from build123d import *

# Parameters (mm, degrees)
BOSS_EXTRUDE1_DEPTH = 3
BOSS_EXTRUDE2_DEPTH = 18
SKETCH3_R           = 12
CUT_EXTRUDE1_DEPTH  = 64.419239983
SKETCH4_R           = 1.6
CUT_EXTRUDE2_DEPTH  = 64.419239983
BOSS_EXTRUDE3_DEPTH = 2
BOSS_EXTRUDE4_DEPTH = 3
SKETCH7_R           = 2.2
CUT_EXTRUDE3_DEPTH  = 63.369864518
SKETCH8_R           = 2.2
CUT_EXTRUDE4_DEPTH  = 63.369864518


with BuildPart() as part:
    # Sketch1 → Boss-Extrude1 (new body)
    with BuildSketch(Plane.XY):
        Polygon((0, -43), (0, 0), (43, 0), (43, -13), (19, -13), (13, -19), (13, -43), align=None)
    extrude(amount=BOSS_EXTRUDE1_DEPTH)

    # Sketch2 → Boss-Extrude2 (add)
    with BuildSketch(Plane.XY.offset(3)):
        Polygon((0, -43), (3, -43), (3, -3), (43, -3), (43, 0), (0, 0), align=None)
    extrude(amount=BOSS_EXTRUDE2_DEPTH)

    # Sketch3 → Cut-Extrude1 (cut, through all)
    with BuildSketch(Plane.XY.offset(3)):
        with Locations((22, -22)):
            Circle(SKETCH3_R)
    extrude(amount=-CUT_EXTRUDE1_DEPTH, mode=Mode.SUBTRACT)

    # Sketch4 → Cut-Extrude2 (cut, through all)
    with BuildSketch(Plane.XY.offset(3)):
        with Locations((6.5, -6.5)):
            Circle(SKETCH4_R)
        with Locations((37.5, -6.5)):
            Circle(SKETCH4_R)
        with Locations((6.5, -37.5)):
            Circle(SKETCH4_R)
    extrude(amount=-CUT_EXTRUDE2_DEPTH, mode=Mode.SUBTRACT)

    # Sketch5 → Boss-Extrude3 (add)
    with BuildSketch(Plane(origin=(43, 0, 0), x_dir=(0, 0, -1), z_dir=(1, 0, 0))):
        Polygon((-3, -10), (-11, -3), (-3, -3), align=None)
    extrude(amount=-BOSS_EXTRUDE3_DEPTH)

    # Sketch6 → Boss-Extrude4 (add)
    with BuildSketch(Plane.XZ.offset(43)):
        Polygon((3, 11), (10, 3), (3, 3), align=None)
    extrude(amount=-BOSS_EXTRUDE4_DEPTH)

    # Sketch7 → Cut-Extrude3 (cut, through all)
    with BuildSketch(Plane.XZ.offset(3)):
        with Locations(Location((13, 11, 0), (0, 0, 270))):
            Circle(SKETCH7_R)
        with Locations(Location((33, 11, 0), (0, 0, 270))):
            Circle(SKETCH7_R)
    extrude(amount=-CUT_EXTRUDE3_DEPTH, mode=Mode.SUBTRACT)

    # Sketch8 → Cut-Extrude4 (cut, through all)
    with BuildSketch(Plane(origin=(3, 0, 0), x_dir=(0, 0, -1), z_dir=(1, 0, 0))):
        with Locations((-11, -33)):
            Circle(SKETCH8_R)
        with Locations((-11, -13)):
            Circle(SKETCH8_R)
    extrude(amount=-CUT_EXTRUDE4_DEPTH, mode=Mode.SUBTRACT)


solid = part.part
Check sheet for the modelled part. Datum: model origin and axes. Units: mm. A direction names the side the tool comes from. Round coordinates to 2 decimals unless told otherwise and drop trailing zeros. Loops run counter-clockwise (first coordinate to the right, second up) from the corner with the lowest first, then second, coordinate; pieces in that order, holes last. Notation, with made-up numbers: (-28, 27) -> (4, 27) arc R32 cw to (4, 58) -> close; hole circle Ø2 at (7.5, -13). An arc over 180 degrees is marked (long way). Put each result on its own line as item: value. Start each with the question number.
1. Section check B-B (z = 2.25). Enter the section's corners in (x, y), plus the area to 3 significant figures.
2. Access from +Z, -Z, +X, -X, +Y, -Y to the whole of each face (thin tool, end or side, straight path). Record for faces 4 (the face through (13, -36, 1)), 5 (the face through (41, -6, 6)), 6 (the face through (42.01, -6.55, 6.94)), 7 (the face through (12.7, -14, 3)).
3. Draft check along Y on faces 1 (the face through (6.45, -41.52, 7.06)), 2 (the face through (37.15, -8.06, 1.52)), 3 (the face through (22, 0, 10)). Enter one of: +Y half, -Y half, draft (parallel to the pull), parting line (faces both ways), or undercut.
4. Section check C-C (x = 37.5). Enter the section's corners in (y, z).
5. Section check D-D (y = -33). Enter the section's corners in (x, z), plus the area to 3 significant figures.
6. Scan lines: probe 1 along Y at (x, z) = (1.3, 11); probe 2 along Y at (x, z) = (37.5, 1.9); probe 3 along X at (y, z) = (-5.5, 8). Record each from-to range of solid material in increasing order.
7. Gauge pin test, flat ends, axial feed: pin 1 (9 mm diameter, centred on x = 22.5, z = 9.5, fed in from -Y); pin 2 (0.9 mm diameter, centred on y = -36, z = 1, fed in from +X); pin 3 (3.5 mm diameter, centred on x = 6.5, y = -37.5, fed in from +Z). Record the tip position at first contact, or that the pin passes through.
8. Section check A-A (y = -6.5). Enter the section's corners in (x, z), plus the area to 3 significant figures.
Findings:
1. outline: (0, -43) -> (13, -43) -> (13, -29.94) arc R12 cw to (29.94, -13) -> (43, -13) -> (43, 0) -> (0, 0) -> close; hole circle Ø3.2 at (6.5, -37.5); hole circle Ø3.2 at (6.5, -6.5); hole circle Ø3.2 at (37.5, -6.5)
1. area: 860 mm^2
2. face 4: +Z, -Z, +X, -Y
2. face 5: +Z, -Y
2. face 6: +Z, +X, -Y
2. face 7: +Z
3. face 1: draft
3. face 2: undercut
3. face 3: +Y half
4. outline: (-13, 0) -> (-8.1, 0) -> (-8.1, 3) -> (-13, 3) -> close; (-4.9, 0) -> (0, 0) -> (0, 21) -> (-3, 21) -> (-3, 3) -> (-4.9, 3) -> close
5. outline: (0, 0) -> (13, 0) -> (13, 3) -> (3, 3) -> (3, 8.8) -> (0, 8.8) -> close; (0, 13.2) -> (3, 13.2) -> (3, 21) -> (0, 21) -> close
5. area: 79.8 mm^2
6. probe 1: y = -43 to -35.2, -30.8 to -15.2, -10.8 to 0
6. probe 2: y = -13 to -8.1, -4.9 to 0
6. probe 3: x = 0 to 3, 41 to 43
7. pin 1: stops at y = -3
7. pin 2: stops at x = 13
7. pin 3: stops at z = 3
8. outline: (0, 0) -> (4.9, 0) -> (4.9, 3) -> (3, 3) -> (3, 21) -> (0, 21) -> close; (8.1, 0) -> (35.9, 0) -> (35.9, 3) -> (8.1, 3) -> close; (39.1, 0) -> (43, 0) -> (43, 7) -> (41, 7) -> (41, 3) -> (39.1, 3) -> close
8. area: 172 mm^2
